Source: CAD feature listing. Evaluate the final solid. Frame: model axes, mm. A direction names the side the tool comes from. Give positions to 0.01 mm unless a question says otherwise; leave off trailing zeros. Loops run counter-clockwise (first coordinate to the right, second up) from the corner with the lowest first, then second, coordinate; pieces in that order, holes last. Notation, with made-up numbers: M 17.25,-26.5 L 34.25,-26.5 A10 cw 34.25,-12.5 Z; hole C 22.5,-15 d10. An arc over 180 degrees is marked long. Answer in a Markdown table with one row per item.
```python
from build123d import *

# Parameters (mm, degrees)
SKETCH_W        = 357
SKETCH_H        = 197
PAD_DEPTH       = 230
SKETCH001_W     = 357
SKETCH001_H     = 230
POCKET_DEPTH    = 5
SKETCH002_W     = 350
SKETCH002_H     = 223
POCKET001_DEPTH = 192
SKETCH003_W     = 165
SKETCH003_H     = 150
POCKET002_DEPTH = 10


with BuildPart() as part:
    # Sketch → Pad (new body)
    with BuildSketch(Plane.XZ):
        with Locations((178.5, 98.5)):
            Rectangle(SKETCH_W, SKETCH_H)
    extrude(amount=PAD_DEPTH)

    # Sketch001 → Pocket (cut)
    with BuildSketch(Plane.XY.offset(192)):
        with Locations((178.5, -115)):
            Rectangle(SKETCH001_W, SKETCH001_H)
    extrude(amount=POCKET_DEPTH, mode=Mode.SUBTRACT)

    # Sketch002 → Pocket001 (cut)
    with BuildSketch(Plane(origin=(3.5, -3.5, 3.5), x_dir=(1, 0, 0), z_dir=(0, 0, 1))):
        with Locations((175, -111.5)):
            Rectangle(SKETCH002_W, SKETCH002_H)
    extrude(amount=POCKET001_DEPTH, mode=Mode.SUBTRACT)

    # Sketch003 → Pocket002 (cut)
    with BuildSketch(Plane(origin=(7.5, -220, 20), x_dir=(1, 0, 0), z_dir=(0, -1, 0))):
        with Locations((82.5, 75)):
            Rectangle(SKETCH003_W, SKETCH003_H)
        with Locations((255.997886, 75)):
            Rectangle(SKETCH003_W, SKETCH003_H)
    extrude(amount=POCKET002_DEPTH, mode=Mode.SUBTRACT)


solid = part.part
```
Q1. Section query B-B (z = 131). Output: boundary loops of the cut face in (x, y).
Values follow:
| item | result |
|---|---|
| outline | M 0,-230 L 7.5,-230 L 7.5,-226.5 L 3.5,-226.5 L 3.5,-3.5 L 353.5,-3.5 L 353.5,-226.5 L 346,-226.5 L 346,-230 L 357,-230 L 357,0 L 0,0 Z; M 172.5,-230 L 181,-230 L 181,-226.5 L 172.5,-226.5 Z |
Q2. Section query A-A (x = 309.5). Output: boundary loops of the cut face in (y, z), plus the area to 3 significant figures.
Values follow:
| item | result |
|---|---|
| outline | M -230,0 L 0,0 L 0,192 L -3.5,192 L -3.5,3.5 L -226.5,3.5 L -226.5,20 L -230,20 Z; M -230,170 L -226.5,170 L -226.5,192 L -230,192 Z |
| area | 1,600 mm^2 |
Q3. Ray query, probe 1 along X at (y, z) = (-98.5, 19.5); probe 2 along Y at (x, z) = (224.5, 175.5); probe 3 along Y at (x, z) = (212, 139). Return the intervals inside material, ascending. Write a range as from..to.
Values follow:
| item | result |
|---|---|
| probe 1 | 0..3.5, 353.5..357 |
| probe 2 | -230..-226.5, -3.5..0 |
| probe 3 | -3.5..0 |
Q4. Contact query for a flat-ended pin moving along its axis: pin 1 Ø1.5 at (x, y) = (140, -68) entering from +Z. Output: stop coordinate, or through.
Values follow:
| item | result |
|---|---|
| pin 1 | z = 3.5 |
Q5. Reachability of faces 5 (the flat face through (176, -113, 3.5)), 6 (the flat face through (0, -113, 95)) from +Z, -Z, +X, -X, +Y, -Y: full face, straight path, thin tool, end or side. Return the list, or none.
Values follow:
| item | result |
|---|---|
| face 5 | +Z |
| face 6 | +Z, -Z, -X, +Y, -Y |
Q6. Mould query, pull axis Y, two halves, no side actions, for faces 1 (the flat face through (178, -226.5, 111)), 2 (the flat face through (353.5, -117, 96)), 3 (the flat face through (178, -230, 104)), 4 (the flat face through (176, -113, 0)). Classes: +Y half, -Y half, draft (parallel to the pull), parting line (faces both ways), or undercut.
Values follow:
| item | result |
|---|---|
| face 1 | undercut |
| face 2 | undercut |
| face 3 | -Y half |
| face 4 | draft |
Q7. Section query C-C (y = -111). Output: boundary loops of the cut face in (x, z), plus the area to 3 significant figures.
Values follow:
| item | result |
|---|---|
| outline | M 0,0 L 357,0 L 357,192 L 353.5,192 L 353.5,3.5 L 3.5,3.5 L 3.5,192 L 0,192 Z |
| area | 2,570 mm^2 |
